Verification items for the finished model (mm, model axes). A direction names the side the tool comes from. Give positions to 0.01 mm unless a question says otherwise; leave off trailing zeros. Loops run counter-clockwise (first coordinate to the right, second up) from the corner with the lowest first, then second, coordinate; pieces in that order, holes last. Notation, with made-up numbers: M 84,49.25 L 105,49.25 A11 ccw 105,61.25 Z; hole C -14,55.5 d7. An arc over 180 degrees is marked long. Use CSV: the item, a comma, the result in double quotes.
from build123d import *

# Parameters (mm, degrees)
EXTRUDE_1_DEPTH      = 3.5
EXTRUDE_1_DEPTH_BACK = 5.5
SKETCH_1_R           = 6
SKETCH_2_W           = 14.3
SKETCH_2_H           = 11.3
EXTRUDE_2_DEPTH      = 13
SKETCH_3_R           = 1.25
EXTRUDE_3_DEPTH      = 1
SKETCH_4_R           = 4.75
EXTRUDE_4_DEPTH      = 11.5
SKETCH_5_R           = 4.25
CUT_EXTRUDE_1_DEPTH  = 11.5
CUT_EXTRUDE_2_REACH  = 102.61


with BuildPart() as part:
    # 草圖1 → 填料-伸長1 (new, two sides: drawn at the far end of the back side and taken through both)
    with BuildSketch(Plane.XY.offset(-EXTRUDE_1_DEPTH_BACK)):
        with Locations((-64.340909091, 31.5)):
            Circle(SKETCH_1_R)
    extrude(amount=EXTRUDE_1_DEPTH + EXTRUDE_1_DEPTH_BACK)

    # 草圖2 → 填料-伸長2 (add)
    with BuildSketch(Plane.XY.offset(3.5)):
        with Locations((-64.340909091, 31.2)):
            Rectangle(SKETCH_2_W, SKETCH_2_H)
    extrude(amount=EXTRUDE_2_DEPTH)

    # 草圖3 → 填料-伸長3 (add)
    with BuildSketch(Plane.XZ.offset(-25.55)):
        with BuildLine():
            Line((-50.690909091, 7.087920564), (-79.690909091, 7.087920564))
            ThreePointArc((-79.690909091, 7.087920564), (-80.751569263, 7.527260393), (-81.190909091, 8.587920564))
            Line((-81.190909091, 8.587920564), (-81.190909091, 48.087920564))
            ThreePointArc((-81.190909091, 48.087920564), (-80.751569263, 49.148580736), (-79.690909091, 49.587920564))
            Line((-79.690909091, 49.587920564), (-50.690909091, 49.587920564))
            ThreePointArc((-50.690909091, 49.587920564), (-49.630248919, 49.148580736), (-49.190909091, 48.087920564))
            Line((-49.190909091, 48.087920564), (-49.190909091, 8.587920564))
            ThreePointArc((-49.190909091, 8.587920564), (-49.630248919, 7.527260393), (-50.690909091, 7.087920564))
        make_face()
        with Locations(Location((-51.190909091, 47.587920564, 0), (0, 0, 270))):
            Circle(SKETCH_3_R, mode=Mode.SUBTRACT)
        with Locations(Location((-79.190909091, 47.587920564, 0), (0, 0, 270))):
            Circle(SKETCH_3_R, mode=Mode.SUBTRACT)
    extrude(amount=EXTRUDE_3_DEPTH)

    # 草圖4 → 填料-伸長4 (add)
    with BuildSketch(Plane(origin=(0, 0, -5.5), x_dir=(-1, 0, 0), z_dir=(0, 0, -1))):
        with Locations((64.340909091, 31.5)):
            Circle(SKETCH_4_R)
    extrude(amount=EXTRUDE_4_DEPTH)

    # 草圖5 → 除料-伸長1 (cut)
    with BuildSketch(Plane(origin=(0, 0, -17), x_dir=(-1, 0, 0), z_dir=(0, 0, -1))):
        with Locations((64.340909091, 31.5)):
            Circle(SKETCH_5_R)
    extrude(amount=-CUT_EXTRUDE_1_DEPTH, mode=Mode.SUBTRACT)

    # 草圖6 → 除料-伸長2 (cut, up to next)
    with BuildSketch(Plane.XY.offset(3.5), mode=Mode.PRIVATE) as cut_extrude_2_sk1:
        with BuildLine():
            Line((-67.057064462, 36.85), (-61.62475372, 36.85))
            ThreePointArc((-61.62475372, 36.85), (-64.340909091, 37.5), (-67.057064462, 36.85))
        make_face()
    cut_extrude_2_tool1 = extrude(cut_extrude_2_sk1.sketch, amount=-CUT_EXTRUDE_2_REACH, mode=Mode.PRIVATE) & part.part
    add(cut_extrude_2_tool1.solids().sort_by_distance((-64.340909, 37.111246, 3.5))[0], mode=Mode.SUBTRACT)


solid = part.part
(1) Section check B-B on x = -76.5. Record the cut outline in (y, z).
Calculated:
outline,"M 24.55,7.09 L 25.55,7.09 L 25.55,49.59 L 24.55,49.59 Z"
(2) Mould release check, pull along X, two halves, no side actions. Record for faces 1 (the cylindrical face through (-80.74, 25.057, 7.516)), 2 (the flat face through (-64, 36.85, 8)), 3 (the flat face through (-64, 32, -5.5)): released by +X, released by -X, zero draft, split by the parting line, or undercut.
Calculated:
face 1,"released by -X"
face 2,"zero draft"
face 3,"undercut"
(3) Section check A-A on y = 31.5. Record the cut outline in (x, z).
Calculated:
outline,"M -71.49,3.5 L -70.34,3.5 L -70.34,-5.5 L -69.09,-5.5 L -69.09,-17 L -68.59,-17 L -68.59,-5.5 L -60.09,-5.5 L -60.09,-17 L -59.59,-17 L -59.59,-5.5 L -58.34,-5.5 L -58.34,3.5 L -57.19,3.5 L -57.19,16.5 L -71.49,16.5 Z"
(4) Section check C-C on z = 34.5. Record the cut outline in (x, y), plus the area to 3 significant figures.
Calculated:
outline,"M -81.19,24.55 L -49.19,24.55 L -49.19,25.55 L -81.19,25.55 Z"
area,"32.0 mm²"
(5) Depth check by flat-ended pin: pin 1 Ø3.5 at (y, z) = (29.5, 11.5) entering from +X; pin 2 Ø4 at (y, z) = (34.5, -7) entering from +X; pin 3 Ø0.5 at (x, y) = (-64.5, 25) entering from -Z; pin 4 Ø6 at (x, z) = (-73.5, -3.5) entering from -Y. Enter the tip coordinate at first touch or a pass-through.
Calculated:
pin 1,"stops at x = -57.19"
pin 2,"stops at x = -58.58"
pin 3,"stops at z = 7.09"
pin 4,"passes through"
(6) Tool access check on faces 4 (the flat face through (-71.491, 31, 10)), 5 (the flat face through (-68, 28, -5.5)), 6 (the flat face through (-64, 31, 16.5)), 7 (the flat face through (-58, 30, 3.5)), 8 (the flat face through (-70.4, 30.4, 3.5)). Record the directions out of +Z, -Z, +X, -X, +Y, -Y that give a thin tool (end or side, any length) a straight path to the whole face; none if there is none.
Calculated:
face 4,"+Z, -Z, -X, +Y"
face 5,"-Z"
face 6,"+Z, +X, -X, +Y"
face 7,"-Z, +X"
face 8,"-Z, -X"
(7) Scan lines: L1, parallel to Z at x = -61, y = 26; L2, parallel to X at y = 29.5, z = -13.5; L3, parallel to Y at x = -67, z = 7. Record each from-to range of solid material in increasing order. Write a range as from..to.
Calculated:
L1,"z = 3.5..16.5"
L2,"x = -68.65..-68.09, -60.59..-60.03"
L3,"y = 25.55..36.85"
